For this review, take the finished solid that the model builds, in its own axes (mm). Give positions to 0.01 mm unless a question says otherwise; leave off trailing zeros. Order: outer loops, then holes, each group sorted by start corner. A loop starts at its lowest first (then second) coordinate and runs counter-clockwise, first axis right, second up. Notation, with made-up numbers: (-36, 51.5) - (14, 51.5) arc R11 ccw to (14, 55.5) - close; hole circle Ø10 at (72.5, 77.25). An arc over 180 degrees is marked (long way). Use a Markdown table: item, result. Add a question column.
1) We need section A-A on y = 0. Write out the cut boundary in (x, z).
2) We need section C-C on z = 11.75. Write out the cut boundary in (x, y), then the cut area to 3 significant figures.
3) We need section B-B on z = 22. Write out the cut boundary in (x, y), then the cut area to 3 significant figures.
4) Wall thickness on L1, parallel to Z at x = -28.5, y = 5; L2, parallel to X at y = -19.5, z = 6.5; L3, parallel to X at y = -18, z = 32.25: over which ranges is each line inside the solid? List them lowest first.
5) Mouldability with a two-part tool opening along X and no side actions: class faces 1 (the face through (-21, -27, 29.566)), 2 (the face through (1, -15, 28.066)), 3 (the face through (-23, 0, 5.176)), 4 (the face through (-51.977, -1.276, 28.414)) as released by +X, released by -X, zero draft, split by the parting line, or undercut.
6) Clearance check with flat-ended pins moving along their axes: P1, Ø1.5, axis at x = -45, z = 11.5, coming from the -Y side; P2, Ø2, axis at x = -6.5, z = 15.5, coming from the -Y side; P3, Ø5, axis at y = 9, z = 23, coming from the -X side. State where each tip first meets the part, or that it passes through.
```python
from build123d import *

# Parameters (mm, degrees)
F2_T = -1.5
F3_R = 3


with BuildPart() as f1:
    # F0 (on Front) → F1 (revolve)
    with BuildSketch(Plane.XZ):
        Polygon((-22.9846419008, 33.67621309), (-22.9846419008, 3.67621309), (-0.4846419008, 3.67621309), (5.0033481255, 28.0664153333), (6.0033481255, 28.0664153333), (6.5153195148, 33.6285006523), align=None)
    revolve(axis=Axis((-22.9846419008, 0, 18.67621309), (0, 0, -1)))

    # F2
    f2_openings = [f1.faces().sort_by_distance(p)[0] for p in [
        (-37.734623, 0, 33.652357),
    ]]
    offset(amount=F2_T, openings=f2_openings, kind=Kind.INTERSECTION)

    # F3
    f3_edges = [f1.edges().sort_by_distance(p)[0] for p in [
        (-44.284651, 0, 5.176213),
    ]]
    fillet(f3_edges, radius=F3_R)


solid = f1.part
```
Checked values:
| question | item | result |
|---|---|---|
| 1 | outline | (-52.48, 33.63) - (-51.97, 28.07) - (-50.97, 28.07) - (-45.48, 3.68) - (-0.48, 3.68) - (5, 28.07) - (6, 28.07) - (6.52, 33.63) - (5.01, 33.63) - (4.64, 29.57) - (3.8, 29.57) - (-1.16, 7.52) arc R3 cw to (-4.08, 5.18) - (-41.88, 5.18) arc R3 cw to (-44.81, 7.52) - (-49.77, 29.57) - (-50.6, 29.57) - (-50.98, 33.63) - close |
| 2 | outline | circle Ø48.63 at (-22.98, 0); hole circle Ø45.56 at (-22.98, 0) |
| 2 | area | 227 mm² |
| 3 | outline | circle Ø53.25 at (-22.98, 0); hole circle Ø50.17 at (-22.98, 0) |
| 3 | area | 250 mm² |
| 4 | L1 | 3.68 to 5.18 |
| 4 | L2 | -35.43 to -31.77, -14.2 to -10.53 |
| 4 | L3 | -46.2 to -44.26, -1.71 to 0.23 |
| 5 | face 1 | undercut |
| 5 | face 2 | zero draft |
| 5 | face 3 | undercut |
| 5 | face 4 | split by the parting line |
| 6 | P1 | y = -11.72 |
| 6 | P2 | y = -19.88 |
| 6 | P3 | x = -49.26 |
